from build123d import *

# Parameters (mm, degrees)
P_IDAT_VYSUNUT_M1_DEPTH  = 14.05
P_IDAT_VYSUNUT_M2_DEPTH  = 1.5
ODEBRAT_VYSUNUT_M1_DEPTH = 1.6
ODEBRAT_VYSUNUT_M2_REACH = 454.909
SKICA4_R                 = 1.5
SKICA5_W                 = 215.84
SKICA5_H                 = 15.55
ODEBRAT_VYSUNUT_M3_DEPTH = 452.805134863


with BuildPart() as part:
    # Skica1 → Přidat vysunutím1 (new body)
    with BuildSketch(Plane.XY):
        Polygon((-1.7, 1.7), (429.98, 1.7), (429.98, -127.624163056), (423.673791129, -133.930371927), (415.733791129, -133.930371927), (413.350841277, -136.313321779), (14.929158723, -136.313321779), (12.546208871, -133.930371927), (4.606208871, -133.930371927), (-1.7, -127.624163056), align=None)
        Polygon((-0.1, 0.1), (428.38, 0.1), (428.38, -126.961421356), (423.01104943, -132.330371927), (415.07104943, -132.330371927), (412.688099577, -134.713321779), (15.591900423, -134.713321779), (13.20895057, -132.330371927), (5.26895057, -132.330371927), (-0.1, -126.961421356), align=None, mode=Mode.SUBTRACT)
    extrude(amount=-P_IDAT_VYSUNUT_M1_DEPTH)

    # Skica2 → Přidat vysunutím2 (add)
    with BuildSketch(Plane.XY):
        Polygon((-1.7, 1.7), (-1.7, -127.624163056), (4.606208871, -133.930371927), (12.546208871, -133.930371927), (14.929158723, -136.313321779), (413.350841277, -136.313321779), (415.733791129, -133.930371927), (423.673791129, -133.930371927), (429.98, -127.624163056), (429.98, 1.7), align=None)
        Polygon((4.3, -4.3), (4.3, -125.138881682), (7.091490245, -127.930371927), (15.031490245, -127.930371927), (17.414440098, -130.313321779), (410.865559902, -130.313321779), (413.248509755, -127.930371927), (421.188509755, -127.930371927), (423.98, -125.138881682), (423.98, -4.3), align=None, mode=Mode.SUBTRACT)
    extrude(amount=P_IDAT_VYSUNUT_M2_DEPTH)

    # Skica3 → Odebrat vysunutím1 (cut)
    with BuildSketch(Plane(origin=(0, 1.7, 0), x_dir=(1, 0, 0), z_dir=(0, 1, 0))):
        with BuildLine():
            Line((45.76, 4.75), (40.26, 4.75))
            ThreePointArc((40.26, 4.75), (36.76, 8.25), (40.26, 11.75))
            Line((40.26, 11.75), (45.76, 11.75))
            ThreePointArc((45.76, 11.75), (49.26, 8.25), (45.76, 4.75))
        make_face()
    extrude(amount=-ODEBRAT_VYSUNUT_M1_DEPTH, mode=Mode.SUBTRACT)

    # Odebrat vysunutím2: up to this face of the body (flat: up to its plane)
    odebrat_vysunut_m2_end = Plane(part.part.faces().sort_by_distance((429.98, -62.962081528, -6.275))[0])
    # Skica4 → Odebrat vysunutím2 (cut, up to the picked face)
    with BuildSketch(Plane.ZY.offset(1.7), mode=Mode.PRIVATE) as odebrat_vysunut_m2_sk1:
        with Locations(Location((-9.05, -22.962081528, 0), (0, 0, 180))):
            Circle(SKICA4_R)
    odebrat_vysunut_m2_tool1 = split(extrude(odebrat_vysunut_m2_sk1.sketch, amount=-ODEBRAT_VYSUNUT_M2_REACH, mode=Mode.PRIVATE), bisect_by=odebrat_vysunut_m2_end, keep=Keep.BOTH, mode=Mode.PRIVATE)
    # Skica4 → Odebrat vysunutím2 (cut, up to the picked face)
    with BuildSketch(Plane.ZY.offset(1.7), mode=Mode.PRIVATE) as odebrat_vysunut_m2_sk2:
        with Locations(Location((-9.05, -102.962081528, 0), (0, 0, 180))):
            Circle(SKICA4_R)
    odebrat_vysunut_m2_tool2 = split(extrude(odebrat_vysunut_m2_sk2.sketch, amount=-ODEBRAT_VYSUNUT_M2_REACH, mode=Mode.PRIVATE), bisect_by=odebrat_vysunut_m2_end, keep=Keep.BOTH, mode=Mode.PRIVATE)
    add(odebrat_vysunut_m2_tool1.solids().sort_by(Axis((-1.7, -22.962082, -9.05), (1, 0, 0)))[0], mode=Mode.SUBTRACT)
    add(odebrat_vysunut_m2_tool2.solids().sort_by(Axis((-1.7, -102.962082, -9.05), (1, 0, 0)))[0], mode=Mode.SUBTRACT)

    # Skica5 → Odebrat vysunutím3 (cut, through all)
    with BuildSketch(Plane(origin=(0, 1.7, 0), x_dir=(1, 0, 0), z_dir=(0, 1, 0))):
        with Locations((322.06, 6.275)):
            Rectangle(SKICA5_W, SKICA5_H)
    extrude(amount=-ODEBRAT_VYSUNUT_M3_DEPTH, mode=Mode.SUBTRACT)


solid = part.part
Check sheet for the modelled part. Datum: model origin and axes. Units: mm. A direction names the side the tool comes from. Round coordinates to 2 decimals unless told otherwise and drop trailing zeros. Write each loop counter-clockwise with the first axis right and the second up, starting at its lowest first coordinate (ties: lowest second). Pieces come first, ordered by that corner, then holes. Notation, with made-up numbers: (-28, 76) - (-2, 76) arc R16 cw to (-2, 92) - close; hole circle Ø11 at (-34, 66.5). An arc over 180 degrees is marked (long way). Return JSON: item names as keys, results as strings.
Q1. Draft check along Y on faces 4 (the flat face through (1.409, -130.733, -6.384)), 5 (the flat face through (214.14, -135, -5)), 6 (the flat face through (75, -2, 0)). Enter one of: released by +Y, released by -Y, zero draft, split by the parting line, or undercut.
Returned:
{"face 4": "released by -Y", "face 5": "zero draft", "face 6": "undercut"}
Q2. Cross-section at C-C (y = -49). Record the boundary of the cut face in (x, z).
Returned:
{"outline": "(-1.7, -14.05) - (-0.1, -14.05) - (-0.1, 0) - (4.3, 0) - (4.3, 1.5) - (-1.7, 1.5) - close"}
Q3. Scan lines: L1, parallel to Y at x = 181.5, z = -10.5; L2, parallel to Y at x = 61.5, z = 0.25; L3, parallel to Y at x = -0.8, z = -9.05. Record each from-to range of solid material in increasing order. Write a range as from..to.
Returned:
{"L1": "y = -136.31..-134.71, 0.1..1.7", "L2": "y = -136.31..-130.31, -4.3..1.7", "L3": "y = -128.52..-104.46, -101.46..-24.46, -21.46..1.7"}
Q4. Cross-section at A-A (x = 188.5). Record the boundary of the cut face in (y, z), then the cut area to 3 significant figures.
Returned:
{"outline": "(-136.31, -14.05) - (-134.71, -14.05) - (-134.71, 0) - (-130.31, 0) - (-130.31, 1.5) - (-136.31, 1.5) - close; (-4.3, 0) - (0.1, 0) - (0.1, -14.05) - (1.7, -14.05) - (1.7, 1.5) - (-4.3, 1.5) - close", "area": "63.0 mm²"}
Q5. Cross-section at B-B (x = 43.5). Record the boundary of the cut face in (y, z), then the cut area to 3 significant figures.
Returned:
{"outline": "(-136.31, -14.05) - (-134.71, -14.05) - (-134.71, 0) - (-130.31, 0) - (-130.31, 1.5) - (-136.31, 1.5) - close; (-4.3, 0) - (0.1, 0) - (0.1, -4.75) - (1.7, -4.75) - (1.7, 1.5) - (-4.3, 1.5) - close; (0.1, -14.05) - (1.7, -14.05) - (1.7, -11.75) - (0.1, -11.75) - close", "area": "51.8 mm²"}
Q6. Access from +Z, -Z, +X, -X, +Y, -Y to the whole of each face (thin tool, end or side, straight path). Record for faces 1 (the flat face through (9, -133.93, -6)), 2 (the flat face through (113, -136.313, -6)), 3 (the flat face through (-0.1, -64, -7)).
Returned:
{"face 1": "+Z, -Z, -X, -Y", "face 2": "+Z, -Z, +X, -X, -Y", "face 3": "-Z, +X"}
Q7. Depth check by flat-ended pin: P1, Ø4, axis at y = -22.96, z = -9.05, coming from the +X side; P2, Ø0.8, axis at y = -79, z = 1, coming from the +X side; P3, Ø6.5, axis at x = 8, z = -6, coming from the -Y side. Enter the tip coordinate at first touch or a pass-through.
Returned:
{"P1": "stops at x = -0.1", "P2": "stops at x = 4.3", "P3": "stops at y = -133.93"}
